Can you work these out from the model? Positions are in its coordinate system, mm. A direction names the side the tool comes from. Give positions to 0.01 mm unless a question says otherwise; leave off trailing zeros. Order: outer loops, then holes, each group sorted by start corner. A loop starts at its lowest first (then second) coordinate and runs counter-clockwise, first axis right, second up. Notation, with made-up numbers: (53, 25.5) - (81, 25.5) arc R31 cw to (81, 60.5) - close; hole circle Ø5 at (75.25, 39.5). An arc over 180 degrees is marked (long way). Answer as a JSON object with one key per item and string values.
```python
from build123d import *

# Parameters (mm, degrees)
SKETCH1_R           = 5
BOSS_EXTRUDE1_DEPTH = 22
BOSS_EXTRUDE2_DEPTH = 67
SKETCH2_R           = 27.5
BOSS_EXTRUDE3_DEPTH = 18
SKETCH5_R           = 14
BOSS_EXTRUDE5_DEPTH = 31
SKETCH6_R           = 12.5
BOSS_EXTRUDE6_DEPTH = 3
SKETCH7_R           = 14
BOSS_EXTRUDE7_DEPTH = 11
SKETCH8_W           = 30
SKETCH8_H           = 67
CUT_EXTRUDE1_DEPTH  = 12.5
SKETCH9_R           = 5
CUT_EXTRUDE2_DEPTH  = 32.5


with BuildPart() as part:
    # Sketch1 → Boss-Extrude1 (new body)
    with BuildSketch(Plane(origin=(0, 0, 0), x_dir=(1, 0, 0), z_dir=(0, 1, 0))):
        with BuildLine():
            Line((0, -30), (51.961524227, -30))
            ThreePointArc((51.961524227, -30), (60, 0), (51.961524227, 30))
            Line((51.961524227, 30), (0, 30))
            Line((0, 30), (-22, 30))
            Line((-22, 30), (-22, 0))
            Line((-22, 0), (-22, -30))
            Line((-22, -30), (0, -30))
        make_face()
        with Locations(Location((30, 0, 0), (0, 0, 270))):
            Circle(SKETCH1_R, mode=Mode.SUBTRACT)
    extrude(amount=BOSS_EXTRUDE1_DEPTH)

    # Sketch1_3 → Boss-Extrude2 (add)
    with BuildSketch(Plane(origin=(0, 0, 0), x_dir=(1, 0, 0), z_dir=(0, 1, 0))):
        Polygon((-44, 30), (-22, 30), (-22, 0), (-22, -30), (-44, -30), align=None)
    extrude(amount=BOSS_EXTRUDE2_DEPTH)

    # Sketch2 → Boss-Extrude3 (add)
    with BuildSketch(Plane.ZY.offset(44)):
        with Locations((0, 37)):
            Circle(SKETCH2_R)
    extrude(amount=BOSS_EXTRUDE3_DEPTH)

    # Sketch3 → Revolve2 (revolve)
    with BuildSketch(Plane.XY, mode=Mode.PRIVATE) as revolve2_sk:
        Polygon((-62, 37), (-74, 37), (-74, 51), (-62, 58), align=None)
    revolve(revolve2_sk.sketch.rotate(Axis((-62, 37, 0), (-1, 0, 0)), 90), axis=Axis((-62, 37, 0), (-1, 0, 0)))

    # Sketch5 → Boss-Extrude5 (add)
    with BuildSketch(Plane.ZY.offset(74)):
        with Locations((0, 37)):
            Circle(SKETCH5_R)
    extrude(amount=BOSS_EXTRUDE5_DEPTH)

    # Sketch6 → Boss-Extrude6 (add)
    with BuildSketch(Plane.ZY.offset(105)):
        with Locations((0, 37)):
            Circle(SKETCH6_R)
    extrude(amount=BOSS_EXTRUDE6_DEPTH)

    # Sketch7 → Boss-Extrude7 (add)
    with BuildSketch(Plane.ZY.offset(108)):
        with Locations((0, 37)):
            Circle(SKETCH7_R)
    extrude(amount=BOSS_EXTRUDE7_DEPTH)

    # Sketch8 → Cut-Extrude1 (cut)
    with BuildSketch(Plane.XY.offset(30)):
        with Locations((-59, 33.5)):
            Rectangle(SKETCH8_W, SKETCH8_H)
    cut_extrude1 = extrude(amount=-CUT_EXTRUDE1_DEPTH, mode=Mode.SUBTRACT)

    # Mirror1: Cut-Extrude1 across plane
    add(cut_extrude1.mirror(Plane.XY), mode=Mode.SUBTRACT)

    # Sketch9 → Cut-Extrude2 (cut)
    with BuildSketch(Plane(origin=(0, 22, 0), x_dir=(1, 0, 0), z_dir=(0, 1, 0))):
        with Locations(Location((0, 0, 0), (0, 0, 270))):
            Circle(SKETCH9_R)
    extrude(amount=-CUT_EXTRUDE2_DEPTH, mode=Mode.SUBTRACT)


solid = part.part
```
Q1. We'd pull the mould along X, two halves only. Please class faces 5 (the face through (-62, 15.8, -0.2)), 6 (the face through (-4.88, 11.15, -1.08)), 7 (the face through (-6, 18, 30)): released by +X, released by -X, zero draft, split by the parting line, or undercut.
Recorded:
{"face 5": "released by -X", "face 6": "undercut", "face 7": "zero draft"}
Q2. If we section it at A-A, the plane z = 0: Count the separate pieces of the cut face and the enclosed holes in it, then the cut area to 3 significant figures.
Recorded:
{"separate pieces": "3", "enclosed holes": "0", "area": "5,500 mm^2"}
Q3. If we section it at D-D, the plane x = -92: Please give me the cut outline in (y, z).
Recorded:
{"outline": "circle Ø28 at (37, 0)"}
Q4. If we section it at C-C, the plane y = 37: Please give me the cut outline in (x, z).
Recorded:
{"outline": "(-119, -14) - (-108, -14) - (-108, -12.5) - (-105, -12.5) - (-105, -14) - (-74, -14) - (-68, -17.5) - (-44, -17.5) - (-44, -30) - (-22, -30) - (-22, 30) - (-44, 30) - (-44, 17.5) - (-68, 17.5) - (-74, 14) - (-105, 14) - (-105, 12.5) - (-108, 12.5) - (-108, 14) - (-119, 14) - close"}
Q5. I need wall thicknesses on L1, parallel to X at y = 7, z = 0; L2, parallel to X at y = 17, z = 0; L3, parallel to X at y = 37.5, z = 1. Which ranges of each line are inside material? Lowest first, please.
Recorded:
{"L1": "x = -44 to -5, 5 to 25, 35 to 60", "L2": "x = -63.71 to -5, 5 to 25, 35 to 60", "L3": "x = -119 to -22"}
Q6. I'm going to push flat-ended pins straight in: pin 1 Ø7 at (x, y) = (-58.5, 37.5) entering from +Z; pin 2 Ø8 at (y, z) = (54, 5) entering from -X; pin 3 Ø5 at (y, z) = (19, -7) entering from -X; pin 4 Ø5 at (x, z) = (-57.5, 20.5) entering from +Y. Where does each tip first touch, or does it pass through?
Recorded:
{"pin 1": "stops at z = 17.5", "pin 2": "stops at x = -119", "pin 3": "stops at x = -69.18", "pin 4": "passes through"}
Q7. Which directions (+Z, -Z, +X, -X, +Y, -Y) give clear straight access to the entire face, cutting with the end or side of a thin tool? Please do faces 1 (the face through (-54, 37, 17.5)), 2 (the face through (-89.28, 23.33, -3.03)), 3 (the face through (-22, 44, 0)), 4 (the face through (-52.9, 9.5, -0.3)).
Recorded:
{"face 1": "+Z, -X, +Y, -Y", "face 2": "-X", "face 3": "+Z, -Z, +X, +Y", "face 4": "-X, -Y"}
Q8. If we section it at B-B, the plane x = 0: Please give me the cut outline in (y, z), then the cut area to 3 significant figures.
Recorded:
{"outline": "(0, -30) - (22, -30) - (22, -5) - (0, -5) - close; (0, 5) - (22, 5) - (22, 30) - (0, 30) - close", "area": "1,100 mm^2"}
